from build123d import *

# Parameters (mm, degrees)
SKETCH_2_R      = 2.55
SKETCH_2_R_2    = 1.1
SKETCH_2_W      = 14
SKETCH_2_H      = 14
SKETCH_2_H_2    = 12
EXTRUDE_1_DEPTH = 5


with BuildPart() as part:
    # 草图2 → 凸台-拉伸1 (new body)
    with BuildSketch(Plane.XY):
        with BuildLine():
            Line((-130, 29.5), (130, 29.5))
            ThreePointArc((130, 29.5), (143.788582233, 23.788582233), (149.5, 10))
            Line((149.5, 10), (149.5, -110))
            ThreePointArc((149.5, -110), (143.788582233, -123.788582233), (130, -129.5))
            Line((130, -129.5), (-130, -129.5))
            ThreePointArc((-130, -129.5), (-143.788582233, -123.788582233), (-149.5, -110))
            Line((-149.5, -110), (-149.5, 10))
            ThreePointArc((-149.5, 10), (-143.788582233, 23.788582233), (-130, 29.5))
        make_face()
        with Locations((130, -110)):
            Circle(SKETCH_2_R, mode=Mode.SUBTRACT)
        with Locations((130, 10)):
            Circle(SKETCH_2_R, mode=Mode.SUBTRACT)
        with Locations((-130, -110)):
            Circle(SKETCH_2_R, mode=Mode.SUBTRACT)
        with Locations((-130, 10)):
            Circle(SKETCH_2_R, mode=Mode.SUBTRACT)
        with Locations((-106, -40)):
            Circle(SKETCH_2_R_2, mode=Mode.SUBTRACT)
        with Locations((-106, -60)):
            Circle(SKETCH_2_R_2, mode=Mode.SUBTRACT)
        with Locations((-16, -40)):
            Circle(SKETCH_2_R_2, mode=Mode.SUBTRACT)
        with Locations((-16, -60)):
            Circle(SKETCH_2_R_2, mode=Mode.SUBTRACT)
        with Locations((-61, -60)):
            Circle(SKETCH_2_R_2, mode=Mode.SUBTRACT)
        with Locations((-61, -40)):
            Circle(SKETCH_2_R_2, mode=Mode.SUBTRACT)
        with Locations(Location((16, -60, 0), (0, 0, 180))):
            Circle(SKETCH_2_R_2, mode=Mode.SUBTRACT)
        with Locations(Location((16, -40, 0), (0, 0, 180))):
            Circle(SKETCH_2_R_2, mode=Mode.SUBTRACT)
        with Locations(Location((61, -60, 0), (0, 0, 180))):
            Circle(SKETCH_2_R_2, mode=Mode.SUBTRACT)
        with Locations(Location((61, -40, 0), (0, 0, 180))):
            Circle(SKETCH_2_R_2, mode=Mode.SUBTRACT)
        with Locations(Location((106, -60, 0), (0, 0, 180))):
            Circle(SKETCH_2_R_2, mode=Mode.SUBTRACT)
        with Locations(Location((106, -40, 0), (0, 0, 180))):
            Circle(SKETCH_2_R_2, mode=Mode.SUBTRACT)
        with Locations((140, -28)):
            Circle(SKETCH_2_R_2, mode=Mode.SUBTRACT)
        with Locations((132, -28)):
            Circle(SKETCH_2_R_2, mode=Mode.SUBTRACT)
        with Locations((132, -72)):
            Circle(SKETCH_2_R_2, mode=Mode.SUBTRACT)
        with Locations((140, -72)):
            Circle(SKETCH_2_R_2, mode=Mode.SUBTRACT)
        with Locations(Location((-140, -72, 0), (0, 0, 180))):
            Circle(SKETCH_2_R_2, mode=Mode.SUBTRACT)
        with Locations(Location((-132, -72, 0), (0, 0, 180))):
            Circle(SKETCH_2_R_2, mode=Mode.SUBTRACT)
        with Locations(Location((-132, -28, 0), (0, 0, 180))):
            Circle(SKETCH_2_R_2, mode=Mode.SUBTRACT)
        with Locations(Location((-140, -28, 0), (0, 0, 180))):
            Circle(SKETCH_2_R_2, mode=Mode.SUBTRACT)
        with Locations((-61, -50)):
            Rectangle(SKETCH_2_W, SKETCH_2_H, mode=Mode.SUBTRACT)
        with Locations((-24, -50)):
            Rectangle(SKETCH_2_W, SKETCH_2_H, mode=Mode.SUBTRACT)
        with Locations((24, -50)):
            Rectangle(SKETCH_2_W, SKETCH_2_H, mode=Mode.SUBTRACT)
        with Locations((136, -87)):
            Rectangle(SKETCH_2_W, SKETCH_2_H, mode=Mode.SUBTRACT)
        with Locations((136, -13)):
            Rectangle(SKETCH_2_W, SKETCH_2_H, mode=Mode.SUBTRACT)
        with BuildLine():
            Line((-20, 12.5), (20, 12.5))
            ThreePointArc((20, 12.5), (26.25, 6.25), (20, 0))
            Line((20, 0), (-20, 0))
            ThreePointArc((-20, 0), (-26.25, 6.25), (-20, 12.5))
        make_face(mode=Mode.SUBTRACT)
        with Locations((-136, -87)):
            Rectangle(SKETCH_2_W, SKETCH_2_H, mode=Mode.SUBTRACT)
        with Locations((-136, -13)):
            Rectangle(SKETCH_2_W, SKETCH_2_H, mode=Mode.SUBTRACT)
        with Locations((-98, -50)):
            Rectangle(SKETCH_2_W, SKETCH_2_H, mode=Mode.SUBTRACT)
        with Locations((61, -50)):
            Rectangle(SKETCH_2_W, SKETCH_2_H, mode=Mode.SUBTRACT)
        with Locations((98, -50)):
            Rectangle(SKETCH_2_W, SKETCH_2_H, mode=Mode.SUBTRACT)
        with Locations((-136, -50)):
            Rectangle(SKETCH_2_W, SKETCH_2_H_2, mode=Mode.SUBTRACT)
        with Locations((136, -50)):
            Rectangle(SKETCH_2_W, SKETCH_2_H_2, mode=Mode.SUBTRACT)
    extrude(amount=EXTRUDE_1_DEPTH)


solid = part.part
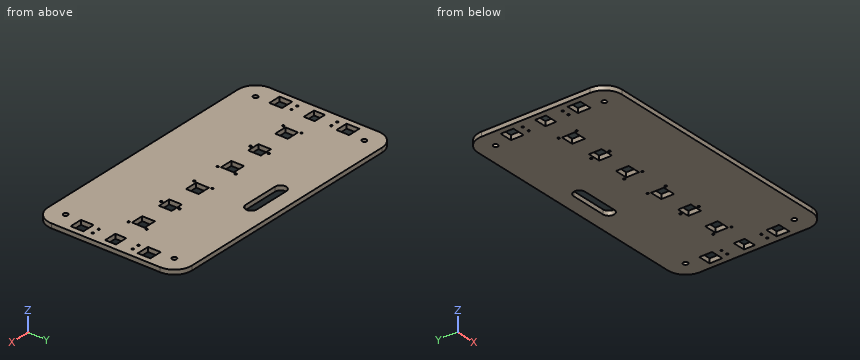
Geometry check sheet. Reference: the model listing, model coordinates, mm. Give positions to 0.01 mm unless a question says otherwise; leave off trailing zeros.
1) Thickness scan on line 1 (X direction, y = -6.5, z = 0.2); line 2 (X direction, y = -72, z = 1.2); line 3 (Y direction, x = -130, z = 3.25). Record the ranges inside material, lowest first.
Values follow:
line 1: x = -149.5 to -143, -129 to 129, 143 to 149.5
line 2: x = -149.5 to -141.1, -138.9 to -133.1, -130.9 to 130.9, 133.1 to 138.9, 141.1 to 149.5
line 3: y = -129.5 to -112.55, -107.45 to -94, -80 to -56, -44 to -20, -6 to 7.45, 12.55 to 29.5
2) Go/stop test with flat-tipped pins: pin 1 Ø3 at (x, y) = (-18.5, -89.5) entering from -Z; pin 2 Ø1.5 at (x, z) = (-132.5, 3.5) entering from -Y; pin 3 Ø1.8 at (x, y) = (132, -28) entering from +Z; pin 4 Ø1.5 at (x, z) = (138, 2) entering from +Y. Record where each tip stops, or that it passes through.
Values follow:
pin 1: stops at z = 0
pin 2: stops at y = -129.42
pin 3: passes through
pin 4: stops at y = 28.1
3) Cross-section at A-A (z = 1.7). Count the separate pieces of the cut face and the enclosed holes in it, plus the area to 3 significant figures.
Values follow:
separate pieces: 1
enclosed holes: 37
area: 44,100 mm2
